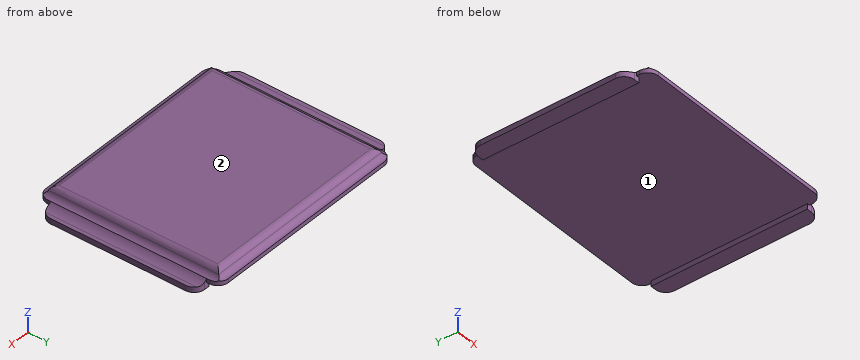
from build123d import *

# Parameters (mm, degrees)
SKETCH1_W             = 0.6
SKETCH1_H             = 5.95
BOSS_EXTRUDE1_DEPTH   = 0.2
BOSS_EXTRUDE1_2_DEPTH = 0.2
BOSS_EXTRUDE2_DEPTH   = 0.15
FILLET1_R             = 0.5
FILLET2_R             = 0.5
SKETCH3_W             = 7.6
SKETCH3_H             = 6.45
BOSS_EXTRUDE3_DEPTH   = 0.3
FILLET3_R             = 0.25
FILLET4_R             = 0.25
FILLET5_R             = 0.25
FILLET6_R             = 0.25
FILLET7_R             = 0.4


# Some blends are built 0.0001 mm under size
with BuildPart() as part:
    # Sketch1 → Boss-Extrude1 (new body)
    with BuildSketch(Plane.XY):
        with Locations((0.3, 2.975)):
            Rectangle(SKETCH1_W, SKETCH1_H)
    extrude(amount=BOSS_EXTRUDE1_DEPTH)



with BuildPart() as body_2:
    # Sketch1 → Boss-Extrude1 2 (new body)
    with BuildSketch(Plane.XY):
        with Locations((8.8, 2.975)):
            Rectangle(SKETCH1_W, SKETCH1_H)
    extrude(amount=BOSS_EXTRUDE1_2_DEPTH)


with BuildPart() as part_1:
    add(part.part)

    add(body_2.part)  # Boss-Extrude2 merges body 2
    # Sketch2 → Boss-Extrude2 (add)
    with BuildSketch(Plane.XY.offset(0.2)):
        Polygon((8.6, 6.45), (8.6, -0.5), (7.9, -0.5), (1.2, -0.5), (0.5, -0.5), (0.5, 6.45), (1.2, 6.45), (7.9, 6.45), align=None)
    extrude(amount=BOSS_EXTRUDE2_DEPTH)

    # Fillet1
    # the kernel refuses this fillet: 0.5 mm, written as the material it adds along each edge
    with BuildSketch(Plane(origin=(0.5, 0, 0.2), x_dir=(-1, 0, 0), z_dir=(0, 1, 0))) as fillet1_piece_1:
        with BuildLine():
            CenterArc((0.357071421, 0.5), FILLET1_R, 224.427004001, 45.572995999)
            Line((0, 0.15), (0, 0))
            Line((0, 0), (0.357071421, 0))
        make_face()
    extrude(amount=5.95)

    # Fillet2
    # the kernel refuses this fillet: 0.5 mm, written as the material it adds along each edge
    with BuildSketch(Plane(origin=(8.6, 5.95, 0.2), x_dir=(0, 0, 1), z_dir=(0, -1, 0))) as fillet2_piece_1:
        with BuildLine():
            CenterArc((0.5, -0.357071421), FILLET2_R, 134.427004001, 45.572995999)
            Line((0, -0.357071421), (0, 0))
            Line((0, 0), (0.15, 0))
        make_face()
    extrude(amount=5.95)

    # Sketch3 → Boss-Extrude3 (add)
    with BuildSketch(Plane.XY.offset(0.35)):
        with Locations((4.55, 2.975)):
            Rectangle(SKETCH3_W, SKETCH3_H)
    extrude(amount=BOSS_EXTRUDE3_DEPTH)

    # Fillet3
    fillet3_edges = [part_1.edges().sort_by_distance(p)[0] for p in [
        (0.75, 2.975, 0.35),
    ]]
    fillet(fillet3_edges, radius=FILLET3_R - 0.0001)  # a hair under: the kernel refuses the full size

    # Fillet4
    fillet4_edges = [part_1.edges().sort_by_distance(p)[0] for p in [
        (8.35, 2.975, 0.35),
    ]]
    fillet(fillet4_edges, radius=FILLET4_R - 0.0001)  # a hair under: the kernel refuses the full size

    # Fillet5
    fillet5_edges = [part_1.edges().sort_by_distance(p)[0] for p in [
        (4.55, 6.2, 0.35),
        (4.55, -0.25, 0.35),
    ]]
    fillet(fillet5_edges, radius=FILLET5_R - 0.0001)  # a hair under: the kernel refuses the full size

    # Fillet6
    fillet6_edges = [part_1.edges().sort_by_distance(p)[0] for p in [
        (8.35, 2.975, 0.65),
        (4.55, 6.2, 0.65),
        (4.55, -0.25, 0.65),
        (0.75, 2.975, 0.65),
    ]]
    fillet(fillet6_edges, radius=FILLET6_R)

    # Fillet7
    # the kernel refuses this fillet: 0.4 mm, written as the material it takes off along each edge
    with BuildSketch(Plane(origin=(9.1, 5.95, -1), x_dir=(-1, 0, 0), z_dir=(0, 0, 1)), Plane(origin=(0, 0, -1), x_dir=(1, 0, 0), z_dir=(0, 0, 1))) as fillet7_piece_1:
        with BuildLine():
            CenterArc((FILLET7_R, FILLET7_R), FILLET7_R, 180, 90)
            Line((0, FILLET7_R), (0, 0))
            Line((0, 0), (FILLET7_R, 0))
        make_face()
    extrude(amount=2.2, mode=Mode.SUBTRACT)
    with BuildSketch(Plane(origin=(8.6, 6.45, -0.8), x_dir=(0, -1, 0), z_dir=(0, 0, 1))) as fillet7_piece_2:
        with BuildLine():
            CenterArc((FILLET7_R, -FILLET7_R), FILLET7_R, 90, 90)
            Line((0, -FILLET7_R), (0, 0))
            Line((0, 0), (FILLET7_R, 0))
        make_face()
    extrude(amount=2.15, mode=Mode.SUBTRACT)
    with BuildSketch(Plane(origin=(8.6, -0.5, -0.8), x_dir=(0, 1, 0), z_dir=(0, 0, 1)), Plane(origin=(0.5, 6.45, -0.8), x_dir=(0, -1, 0), z_dir=(0, 0, 1)), Plane(origin=(0.5, -0.5, -0.8), x_dir=(1, 0, 0), z_dir=(0, 0, 1))) as fillet7_piece_3:
        with BuildLine():
            CenterArc((FILLET7_R, FILLET7_R), FILLET7_R, 180, 90)
            Line((0, FILLET7_R), (0, 0))
            Line((0, 0), (FILLET7_R, 0))
        make_face()
    extrude(amount=2.15, mode=Mode.SUBTRACT)
    with BuildSketch(Plane(origin=(9.1, 0, -1), x_dir=(-1, 0, 0), z_dir=(0, 0, 1)), Plane(origin=(0, 5.95, -1), x_dir=(1, 0, 0), z_dir=(0, 0, 1))) as fillet7_piece_4:
        with BuildLine():
            CenterArc((FILLET7_R, -FILLET7_R), FILLET7_R, 90, 90)
            Line((0, -FILLET7_R), (0, 0))
            Line((0, 0), (FILLET7_R, 0))
        make_face()
    extrude(amount=2.2, mode=Mode.SUBTRACT)


solid = part_1.part
Geometry check sheet. Reference: the model listing, model coordinates, mm. Face numbers are marked on the shaded views. Give positions to 0.01 mm unless a question says otherwise; leave off trailing zeros. Write each loop counter-clockwise with the first axis right and the second up, starting at its lowest first coordinate (ties: lowest second). Pieces come first, ordered by that corner, then holes. Notation, with made-up numbers: (11, -9.5) - (29, -9.5) arc R31 ccw to (29, 24.5) - close; hole circle Ø6 at (48, 8.25). An arc over 180 degrees is marked (long way). Put each result on its own line as item: value.
1. Sectioned sample at A-A, the plane z = 0.1. Enter the section's corners in (x, y).
Ans:
outline: (0, 0.4) arc R0.4 ccw to (0.4, 0) - (0.6, 0) - (0.6, 5.95) - (0.4, 5.95) arc R0.4 ccw to (0, 5.55) - close; (8.5, 0) - (8.7, 0) arc R0.4 ccw to (9.1, 0.4) - (9.1, 5.55) arc R0.4 ccw to (8.7, 5.95) - (8.5, 5.95) - close
2. Thickness scan on line 1 (X direction, y = 1.5, z = 0.1); line 2 (Z direction, x = 6.75, y = 0); line 3 (Y direction, x = 5.75, z = 0.5). Record the ranges inside material, lowest first.
Ans:
line 1: x = 0 to 0.6, 8.5 to 9.1
line 2: z = 0.2 to 0.65
line 3: y = -0.27 to 6.22
3. Draft check along X on the marked faces 1 and 2. Enter one of: +X half, -X half, draft (parallel to the pull), parting line (faces both ways), or undercut.
Ans:
face 1: undercut
face 2: draft
